Could you check a few things on this model? Use its own coordinates, in mm. Face numbers are marked on the shaded views. Give positions to 0.01 mm unless a question says otherwise; leave off trailing zeros. Loops run counter-clockwise (first coordinate to the right, second up) from the corner with the lowest first, then second, coordinate; pieces in that order, holes last. Notation, with made-up numbers: M 26,-4.5 L 52,-4.5 A17 cw 52,11.5 Z; hole C 72,48.25 d7. An arc over 180 degrees is marked long. Return JSON: item names as keys, results as strings. Group by question number.
1. For pin 1 (10 mm diameter, centred on x = -4.5, z = 27.5, fed in from +Y); pin 2 (10 mm diameter, centred on y = -6, z = 25, fed in from +X); pin 3 (6 mm diameter, centred on x = 1.5, z = 13.5, fed in from +Y), each with a flat end and sliding along its axis, tell me the tip position at first contact or that it passes through.
2. If we section it at A-A (x = 0): Write out the boundary of the cut face in (y, z), plus the area to 3 significant figures.
3. If we mould it in two halves opening along Y, with no side actions, what happens to the marked faces 1 and 2? For each: +Y half, -Y half, draft (parallel to the pull), parting line (faces both ways), or undercut.
4. If we section it at D-D (z = 22.5): Write out the boundary of the cut face in (x, y) (3 decimals).
5. Please list where these lines run through material, in increasing order: line 1 (Y direction, x = 5.25, z = 14.5); line 2 (X direction, y = -0.25, z = 30.5); line 3 (X direction, y = 7, z = 20).
6. If we section it at C-C (z = 10): Write out the boundary of the cut face in (x, y), plus the area to 3 significant figures.
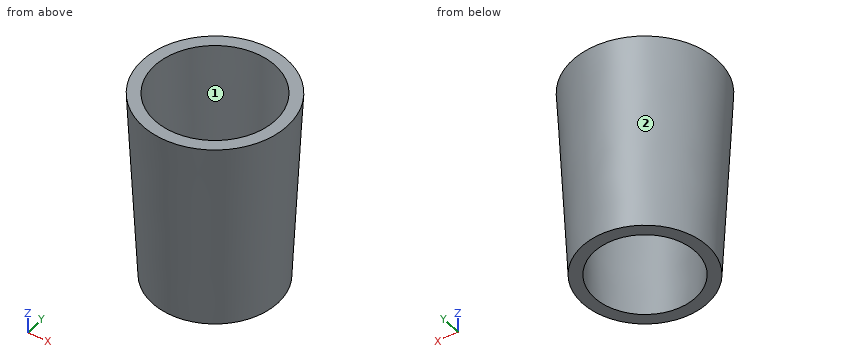
```python
from build123d import *


with BuildPart() as cone001:
    # Cone001 → Cone001 (revolve)
    with BuildSketch(Plane.XZ):
        Polygon((0, 0), (8.4, 0), (10, 32), (0, 32), align=None)
    revolve(axis=Axis((0, 0, 0), (0, 0, 1)))


with BuildPart() as obj1:
    # Cone002 → Cone002 (revolve)
    with BuildSketch(Plane(origin=(0, 0, 2), x_dir=(1, 0, 0), z_dir=(0, -1, 0))):
        Polygon((0, 0), (10.5, 0), (11.9, 28), (0, 28), align=None)
    revolve(axis=Axis((0, 0, 2), (0, 0, 1)))


with BuildPart() as is383_joint:
    # Cone → Cone (revolve)
    with BuildSketch(Plane.XZ):
        Polygon((0, 0), (10.4, 0), (12, 32), (0, 32), align=None)
    revolve(axis=Axis((0, 0, 0), (0, 0, 1)))

    # Fusion: union obj1
    add(obj1.part)

    # Cut: cut Cone001
    add(cone001.part, mode=Mode.SUBTRACT)


solid = is383_joint.part
```
Answer:
{
 "1": {"pin 1": "stops at y = 11.92", "pin 2": "stops at x = 11.66", "pin 3": "stops at y = 11.21"},
 "2": {"outline": "M -12,32 L -10.4,0 L -8.4,0 L -10,32 Z; M 8.4,0 L 10.4,0 L 12,32 L 10,32 Z", "area": "128 mm²"},
 "3": {"face 1": "undercut", "face 2": "parting line"},
 "4": {"outline": "C 0,0 d23.05; hole C 0,0 d19.05"},
 "5": {"line 1": "y = -9.81 to -7.46, 7.46 to 9.81", "line 2": "x = -11.92 to -9.92, 9.92 to 11.92", "line 3": "x = -9 to -6.27, 6.27 to 9"},
 "6": {"outline": "C 0,0 d21.8; hole C 0,0 d17.8", "area": "124 mm²"}
}
